```python
from build123d import *

# Parameters (mm, degrees)
F0_R          = 11
F1_DEPTH      = 18
F3_DEPTH      = 8
F4_R          = 4.225
F5_DEPTH      = 8
F6_R          = 1.6
F7_DEPTH      = 25
F7_DEPTH_BACK = 25
F9_START      = 5
F9_DEPTH      = 3.5
F10_START     = -5
F10_DEPTH     = 3.5


with BuildPart() as f1:
    # F0 (on Top) → F1 (new body)
    with BuildSketch(Plane.XY):
        Circle(F0_R)
    extrude(amount=F1_DEPTH)

    # F2 (on face) → F3 (cut)
    with BuildSketch(Plane(origin=(0, 0, 0), x_dir=(1, 0, 0), z_dir=(0, 0, -1))):
        with BuildLine():
            Line((1.7146428199, 2.15), (-1.7146428199, 2.15))
            ThreePointArc((-1.7146428199, 2.15), (0, -2.75), (1.7146428199, 2.15))
        make_face()
    extrude(amount=-F3_DEPTH, mode=Mode.SUBTRACT)

    # F4 (on face) + F0 (on Top) → F5 (cut)
    with BuildSketch(Plane.XY.offset(18)):
        Circle(F4_R)
    with BuildSketch(Plane.XY):
        Circle(F0_R)
    extrude(amount=-F5_DEPTH, mode=Mode.SUBTRACT)

    # F6 (on Front) → F7 (cut, two sides)
    with BuildSketch(Plane.XZ) as f7_sk:
        with Locations((0, 4)):
            Circle(F6_R)
        with Locations((0, 14)):
            Circle(F6_R)
    extrude(amount=F7_DEPTH, mode=Mode.SUBTRACT)
    extrude(f7_sk.sketch, amount=-F7_DEPTH_BACK, mode=Mode.SUBTRACT)

    # F8 (on Front) → F9 (cut)
    with BuildSketch(Plane.XZ.offset(F9_START)):
        Polygon((-3, 5.7320508076), (-3, 2.2679491924), (-3, -7.7320508076), (3, -7.7320508076), (3, 2.2679491924), (3, 5.7320508076), (0, 7.4641016151), align=None)
        Polygon((-3, 15.7320508076), (-3, 12.2679491924), (0, 10.5358983849), (3, 12.2679491924), (3, 15.7320508076), (3, 25.7320508076), (-3, 25.7320508076), align=None)
    extrude(amount=F9_DEPTH, mode=Mode.SUBTRACT)

    # F8 (on Front) → F10 (cut)
    with BuildSketch(Plane.XZ.offset(F10_START)):
        Polygon((-3, 5.7320508076), (-3, 2.2679491924), (-3, -7.7320508076), (3, -7.7320508076), (3, 2.2679491924), (3, 5.7320508076), (0, 7.4641016151), align=None)
        Polygon((-3, 15.7320508076), (-3, 12.2679491924), (0, 10.5358983849), (3, 12.2679491924), (3, 15.7320508076), (3, 25.7320508076), (-3, 25.7320508076), align=None)
    extrude(amount=-F10_DEPTH, mode=Mode.SUBTRACT)


solid = f1.part
```
For this review, take the finished solid that the model builds, in its own axes (mm). A direction names the side the tool comes from. Round coordinates to 2 decimals unless told otherwise and drop trailing zeros. Write each loop counter-clockwise with the first axis right and the second up, starting at its lowest first coordinate (ties: lowest second). Pieces come first, ordered by that corner, then holes.
1) Take a section at C-C on y = -9.25. Give the boundary of the cut face in (x, z).
Answer below:
outline: (-5.95, 0) - (5.95, 0) - (5.95, 18) - (-5.95, 18) - close; hole circle Ø3.2 at (0, 4); hole circle Ø3.2 at (0, 14)
2) Machinability: for faces 5 (the face through (-0.35, -3.56, 2.44)), 6 (the face through (-3, 7, 15)), 7 (the face through (-1.5, -6.7, 6.6)), which of the approach directions +Z, -Z, +X, -X, +Y, -Y give a long, thin tool a straight path to every point of the face, cutting with its end or side? Answer none if there is none.
Answer below:
face 5: +Y, -Y
face 6: +Z
face 7: -Z
3) Mouldability with a two-part tool opening along Z and no side actions: class faces 1 (the face through (-0.35, 9.73, 2.44)), 2 (the face through (1.5, 6.7, 11.4)), 3 (the face through (1.5, 6.7, 6.6)), 4 (the face through (0, 5, 16)) as +Z half, -Z half, draft (parallel to the pull), parting line (faces both ways), or undercut.
Answer below:
face 1: undercut
face 2: +Z half
face 3: -Z half
face 4: draft
4) Take a section at B-B on z = 11.75. Give the boundary of the cut face in (x, y) (3 decimals), then the cut area to 3 significant figures.
Answer below:
outline: circle Ø22 at (0, 0); hole circle Ø8.45 at (0, 0); hole (-2.103, -8.5) - (2.103, -8.5) - (2.103, -5) - (-2.103, -5) - close; hole (-2.103, 5) - (2.103, 5) - (2.103, 8.5) - (-2.103, 8.5) - close
area: 295 mm2
5) For line 1 along Z through (x, y) = (0, 9.25); line 2 along Z through (x, y) = (0, 3.4); line 3 along Y through (x, z) = (-2, 5), list the stretches that pass through material, from the lowest coordinate up.
Answer below:
line 1: z = 0 to 2.4, 5.6 to 12.4, 15.6 to 18
line 2: z = 0 to 2.4, 5.6 to 10
line 3: y = -10.82 to -8.5, -5 to -1.89, 1.89 to 5, 8.5 to 10.82
6) Take a section at D-D on y = 1. Give the boundary of the cut face in (x, z), then the cut area to 3 significant figures.
Answer below:
outline: (-10.95, 0) - (-2.56, 0) - (-2.56, 8) - (2.56, 8) - (2.56, 0) - (10.95, 0) - (10.95, 18) - (4.1, 18) - (4.1, 10) - (-4.1, 10) - (-4.1, 18) - (-10.95, 18) - close
area: 288 mm2
7) Take a section at A-A on z = 15. Give the boundary of the cut face in (x, y) (3 decimals), then the cut area to 3 significant figures.
Answer below:
outline: (-3, -8.5) - (-3, -5) - (-1.249, -5) - (-1.249, -4.036) arc R4.225 cw to (-1.249, 4.036) - (-1.249, 5) - (-3, 5) - (-3, 8.5) - (-1.249, 8.5) - (-1.249, 10.929) arc R11 ccw to (-1.249, -10.929) - (-1.249, -8.5) - close; (1.249, -10.929) arc R11 ccw to (1.249, 10.929) - (1.249, 8.5) - (3, 8.5) - (3, 5) - (1.249, 5) - (1.249, 4.036) arc R4.225 cw to (1.249, -4.036) - (1.249, -5) - (3, -5) - (3, -8.5) - (1.249, -8.5) - close
area: 265 mm2
8) Insertion check: pin 1 Ø3 at (x, z) = (-4, 13) entering from -Y; pin 2 Ø3 at (y, z) = (-6.5, 16) entering from -X; pin 3 Ø3.5 at (x, y) = (0, 0) entering from +Z; pin 4 Ø2.5 at (x, z) = (0, 14) entering from +Y. Each pin has a flat end and moves straight along its axis. Give the tip position at first contact, or say it passes through.
Answer below:
pin 1: stops at y = -10.71
pin 2: stops at x = -9.8
pin 3: stops at z = 10
pin 4: passes through
